Answer from the drawing. Dimensions are ordinates in mm from the lowest x, y and z of the part. A direction names the side the tool comes from. Round coordinates to 2 decimals unless told otherwise and drop trailing zeros. Loops run counter-clockwise (first coordinate to the right, second up) from the corner with the lowest first, then second, coordinate; pieces in that order, holes last. Notation, with made-up numbers: M -14.75,-18.75 L 29.25,-18.75 A22 cw 29.25,3.25 Z; hole C 34,50.5 d10. An arc over 180 degrees is marked long. Write each question's results on one line, items separated by ' | '.
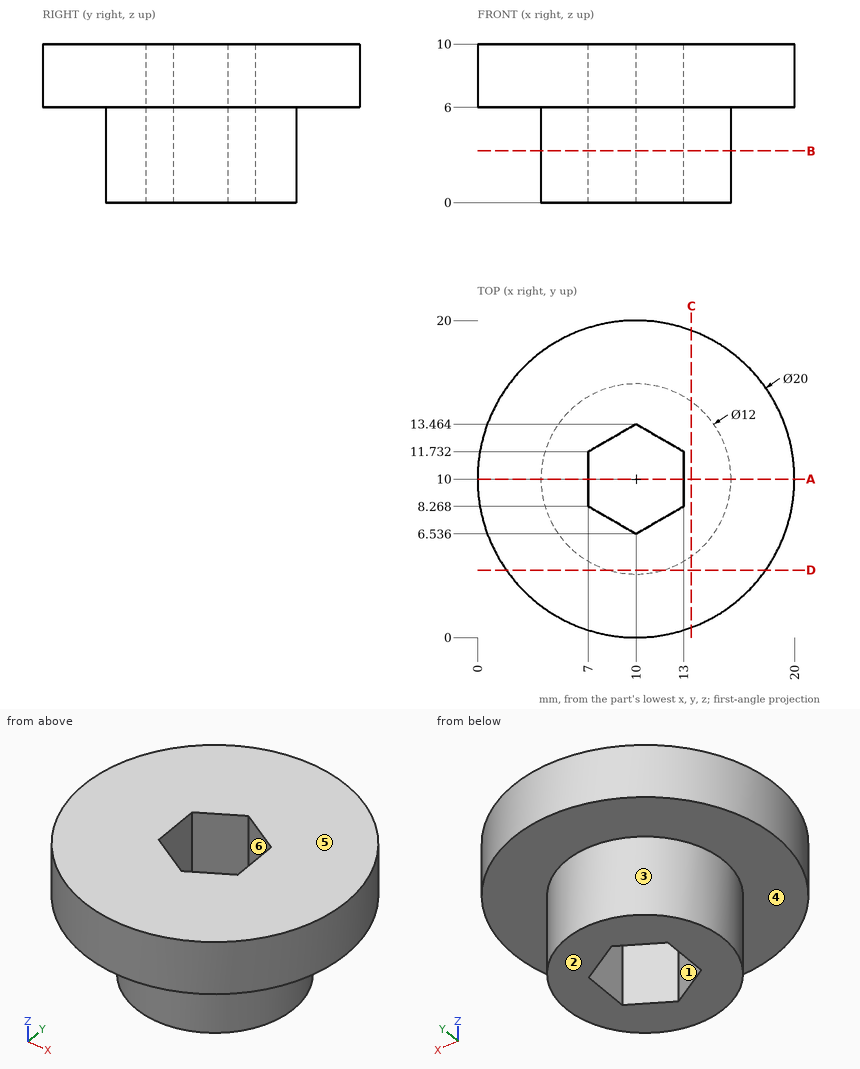
1. Given P1, Ø8, axis at x = 2, y = 17, coming from the -Z side; P2, Ø10, axis at x = 9.5, y = 7.5, coming from the -Z side; P3, Ø2, axis at y = 10.5, z = 1.5, coming from the +X side; P4, Ø3, axis at y = 9.5, z = 3.5, coming from the -X side, each flat-ended and moving along its own axis, determine where each tip first touches the part or whether it passes through.
Completed:
P1: stops at z = 6 | P2: stops at z = 0 | P3: stops at x = 16 | P4: stops at x = 4
2. Find section B-B, the plane z = 3.25. Give the vertices of the cut face in (x, y), then the cut area to 3 significant figures.
Completed:
outline: C 10,10 d12; hole M 7,8.27 L 10,6.54 L 13,8.27 L 13,11.73 L 10,13.46 L 7,11.73 Z | area: 81.9 mm2
3. Find section A-A, the plane y = 10. Give the vertices of the cut face in (x, z).
Completed:
outline: M 0,6 L 4,6 L 4,0 L 7,0 L 7,10 L 0,10 Z; M 13,0 L 16,0 L 16,6 L 20,6 L 20,10 L 13,10 Z
4. Find section C-C, the plane x = 13.5. Give the vertices of the cut face in (y, z).
Completed:
outline: M 0.63,6 L 5.13,6 L 5.13,0 L 14.87,0 L 14.87,6 L 19.37,6 L 19.37,10 L 0.63,10 Z
5. Which of the six approach directions +Z, -Z, +X, -X, +Y, -Y give full straight-line access (tool end or side, diameter ignored) to the marked faces 4, 5 and 6?
Completed:
face 4: -Z | face 5: +Z, +X, -X, +Y, -Y | face 6: +Z, -Z
6. Find section D-D, the plane y = 4.25. Give the vertices of the cut face in (x, z), then the cut area to 3 significant figures.
Completed:
outline: M 1.82,6 L 8.29,6 L 8.29,0 L 11.71,0 L 11.71,6 L 18.18,6 L 18.18,10 L 1.82,10 Z | area: 86.0 mm2
7. Find the intervals of material crossed by L1, parallel to Z at x = 14.25, y = 4.5; L2, parallel to Y at x = 9.5, z = 4.25 (1 decimal); L3, parallel to Y at x = 7.75, z = 9.75 (1 decimal), in increasing order.
Completed:
L1: z = 6 to 10 | L2: y = 4 to 6.8, 13.2 to 16 | L3: y = 0.3 to 7.8, 12.2 to 19.7
8. Determine the mould class of the marked faces 1, 2 and 3 for opening direction Y: released by +Y, released by -Y, zero draft, split by the parting line, or undercut.
Completed:
face 1: undercut | face 2: zero draft | face 3: split by the parting line
